Check sheet for the modelled part. Datum: model origin and axes. Units: mm. A direction names the side the tool comes from. Coordinates: 2 decimals unless noted, no trailing zeros. Loops run counter-clockwise (first coordinate to the right, second up) from the corner with the lowest first, then second, coordinate; pieces in that order, holes last. Notation, with made-up numbers: (76.5, 21.5) -> (118.5, 21.5) arc R11 cw to (118.5, 25.5) -> close; hole circle Ø11 at (85.25, 39.25). An arc over 180 degrees is marked (long way). Use CSV: the item, a comma, the result in double quotes. Start each with the question number.
1. Sectioned sample at B-B, the plane z = 5.5. Record the cut outline in (x, y).
2. Gauge pin test, flat ends, axial feed: pin 1 (3 mm diameter, centred on x = -18, z = 19.5, fed in from -Y); pin 2 (6 mm diameter, centred on y = -15.5, z = 20, fed in from +X); pin 3 (4.5 mm diameter, centred on y = -25, z = 16.5, fed in from -X); pin 4 (1.5 mm diameter, centred on x = -9, z = 11, fed in from -Y). Record the tip position at first contact, or that the pin passes through.
3. Sectioned sample at C-C, the plane y = -23.5. Record the cut outline in (x, z).
4. Thickness scan on L1, parallel to X at y = 23, z = 6.75; L2, parallel to Y at x = -16.25, z = 21.75; L3, parallel to Y at x = -14.25, z = 21.5. Record the ranges inside material, lowest first.
5. Set-up check for faces 5 (the face through (-5, -25, 12)), 6 (the face through (0, 23, 12)): record each of +Z, -Z, +X, -X, +Y, -Y from which the full face is reachable in a straight line by a thin tool's end or side.
6. Release check for a two-part mould opening along Y. For faces 1 (the face through (-2, -27.5, 12)), 2 (the face through (-22.496, -0.424, 12.325)), 3 (the face through (-5, 25, 12)), 4 (the face through (-17.496, 0.385, 12.325)) record: pulls with the +Y half, pulls with the -Y half, needs draft (parallel to the pull), parting line crosses it, or undercut.
7. Sectioned sample at A-A, the plane x = -4. Record the cut outline in (y, z), and give its area (3 significant figures).
8. Sectioned sample at D-D, the plane x = -12.75. Record the cut outline in (y, z), and give its area (3 significant figures).
```python
from build123d import *

# Parameters (mm, degrees)
BOSS_EXTRUDE1_DEPTH = 25


with BuildPart() as part:
    # Sketch4 → Boss-Extrude1 (new body)
    with BuildSketch(Plane.XY):
        with BuildLine():
            Line((0, 22.5), (0, 17.5))
            ThreePointArc((0, 17.5), (-17.5, 0), (0, -17.5))
            Line((0, -17.5), (0, -22.5))
            Line((0, -22.5), (0, -27.5))
            Line((0, -27.5), (-5, -27.5))
            Line((-5, -27.5), (-5, -22.5))
            Line((-5, -22.5), (-5, -21.937410968))
            ThreePointArc((-5, -21.937410968), (-22.5, 0), (-5, 21.937410968))
            Line((-5, 21.937410968), (-5, 22.5))
            Line((-5, 22.5), (-5, 27.5))
            Line((-5, 27.5), (0, 27.5))
            Line((0, 27.5), (0, 22.5))
        make_face()
    extrude(amount=BOSS_EXTRUDE1_DEPTH)


solid = part.part
```
Completed:
1,outline,"(-5, -27.5) -> (0, -27.5) -> (0, -17.5) arc R17.5 cw to (0, 17.5) -> (0, 27.5) -> (-5, 27.5) -> (-5, 21.94) arc R22.5 ccw to (-5, -21.94) -> close"
2,pin 1,"y = -15.3"
2,pin 2,"x = 0"
2,pin 3,"x = -5"
2,pin 4,"y = -20.93"
3,outline,"(-5, 0) -> (0, 0) -> (0, 25) -> (-5, 25) -> close"
4,L1,"-5 to 0"
4,L2,"-15.56 to -6.5, 6.5 to 15.56"
4,L3,"-17.41 to -10.16, 10.16 to 17.41"
5,face 5,"+Z, -Z, -X, -Y"
5,face 6,"+Z, -Z, +X, +Y, -Y"
6,face 1,"pulls with the -Y half"
6,face 2,"parting line crosses it"
6,face 3,"needs draft"
6,face 4,"undercut"
7,outline,"(-27.5, 0) -> (-17.04, 0) -> (-17.04, 25) -> (-27.5, 25) -> close; (17.04, 0) -> (27.5, 0) -> (27.5, 25) -> (17.04, 25) -> close"
7,area,"523 mm²"
8,outline,"(-18.54, 0) -> (-11.99, 0) -> (-11.99, 25) -> (-18.54, 25) -> close; (11.99, 0) -> (18.54, 0) -> (18.54, 25) -> (11.99, 25) -> close"
8,area,"328 mm²"
